from build123d import *

# Parameters (mm, degrees)
F0_R     = 4.5
F1_DEPTH = 7.62
F3_DEPTH = 7.62


with BuildPart() as f1:
    # F0 (on Top) → F1 (new body)
    with BuildSketch(Plane.XY):
        Polygon((-46.3863605133, -12.5119441933), (30.6131504527, -12.5119441933), (41.8083587594, -12.5119441933), (41.8083587594, 80.9429615394), (21.555083004, 80.9429615394), (-37.3282930646, 80.9429615394), (-57.58156882, 80.9429615394), (-57.58156882, -12.5119441933), align=None)
        with Locations((-42.3521250486, -5.9729921632)):
            Circle(F0_R, mode=Mode.SUBTRACT)
        Polygon((-27.3236659841, -8.2207562408), (-15.2949382399, -5.5129789378), (-0.4782718207, -5.5129789378), (11.5504559235, -8.2207562408), align=None, mode=Mode.SUBTRACT)
        with Locations((26.578914988, -5.9729921632)):
            Circle(F0_R, mode=Mode.SUBTRACT)
        Polygon((-25.793466622, 41.4102652967), (-25.793466622, 19.9220313867), (-53.3758333607, -8.2207562408), (-53.3758333607, 76.8635385285), (-25.793466622, 50.1095634738), align=None, mode=Mode.SUBTRACT)
        with Locations((-42.3521250486, 75.2675160766)):
            Circle(F0_R, mode=Mode.SUBTRACT)
        Polygon((-31.369628484, 76.8635385285), (15.5964184234, 76.8635385285), (-7.8866050303, 60.7865828711), align=None, mode=Mode.SUBTRACT)
        Polygon((37.6026233001, -8.2207562408), (10.0202565614, 19.9220313867), (10.0202565614, 41.4102652967), (10.0202565614, 50.1095634738), (37.6026233001, 76.8635385285), align=None, mode=Mode.SUBTRACT)
        with Locations((26.578914988, 75.2675160766)):
            Circle(F0_R, mode=Mode.SUBTRACT)
    extrude(amount=F1_DEPTH)

    # F2 (on face) → F3 (join)
    with BuildSketch(Plane.XY.offset(7.62)):
        Polygon((-7.8866050303, 60.7865828711), (-25.793466622, 50.1095634738), (-25.793466622, 19.9220313867), (-25.793466622, 6.6224359907), (-7.8866050303, -5.5129789378), (10.0202565614, 6.6224359907), (10.0202565614, 19.9220313867), (10.0202565614, 50.1095634738), align=None)
        Polygon((-21.9546725898, 45.3533753753), (-7.8866050303, 56.6663203104), (6.1814625292, 45.3533753753), (6.1814625292, 11.3457208499), (-7.8866050303, 0), (-21.9546725898, 11.3457208499), align=None, mode=Mode.SUBTRACT)
    extrude(amount=F3_DEPTH)


solid = f1.part
Geometry: final body of the model. Coordinates: model frame, mm. A direction names the side the tool comes from. Give positions to 0.01 mm unless a question says otherwise; leave off trailing zeros. Order: outer loops, then holes, each group sorted by start corner. A loop starts at its lowest first (then second) coordinate and runs counter-clockwise, first axis right, second up. Notation, with made-up numbers: (-30, -0.5) -> (27, -0.5) arc R10 cw to (27, 18.5) -> close; hole circle Ø2 at (40, -13). An arc over 180 degrees is marked (long way). Put each result on its own line as item: value.
Q1. Section C-C, the plane z = 13.5. Return loops of the section in (x, y).
Here are the results:
outline: (-25.79, 6.62) -> (-7.89, -5.51) -> (10.02, 6.62) -> (10.02, 50.11) -> (-7.89, 60.79) -> (-25.79, 50.11) -> close; hole (-21.95, 11.35) -> (-7.89, 0) -> (6.18, 11.35) -> (6.18, 45.35) -> (-7.89, 56.67) -> (-21.95, 45.35) -> close
Q2. Section D-D, the plane x = -13. Return loops of the section in (y, z), then the cut area to 3 significant figures.
Here are the results:
outline: (-12.51, 0) -> (-8.22, 0) -> (-8.22, 7.62) -> (-12.51, 7.62) -> close; (-5.51, 0) -> (64.29, 0) -> (64.29, 7.62) -> (57.74, 7.62) -> (57.74, 15.24) -> (52.55, 15.24) -> (52.55, 7.62) -> (4.12, 7.62) -> (4.12, 15.24) -> (-2.05, 15.24) -> (-2.05, 7.62) -> (-5.51, 7.62) -> close; (76.86, 0) -> (80.94, 0) -> (80.94, 7.62) -> (76.86, 7.62) -> close
area: 682 mm^2
Q3. Reachability of faces 1 (the face through (6.181, 29, 11)), 2 (the face through (0.94, 0.47, 11.38)), 3 (the face through (41.808, 34, 4)), 4 (the face through (-19.46, 68.71, 3.76)) from +Z, -Z, +X, -X, +Y, -Y: full face, straight path, thin tool, end or side. Return the list, or none.
Here are the results:
face 1: +Z
face 2: +Z, +X, -Y
face 3: +Z, -Z, +X, +Y, -Y
face 4: +Z, -Z
Q4. Draft query along X for faces 5 (the face through (-7, 80.943, 4)), 6 (the face through (-16.715, 55.523, 11.377)), 7 (the face through (37.603, 35, 4)), 8 (the face through (-53.376, 34, 4)). Return one class per face: released by +X, released by -X, zero draft, split by the parting line, or undercut.
Here are the results:
face 5: zero draft
face 6: released by -X
face 7: undercut
face 8: undercut
Q5. Pin query (flat end, axial travel): pin 1 (11.5 mm diameter, centred on x = -42.35, y = 75.27, fed in from +Z); pin 2 (5.5 mm diameter, centred on x = -42.35, y = -5.97, fed in from -Z); pin 3 (1 mm diameter, centred on x = -10, z = 9.5, fed in from -Y); pin 4 (8.5 mm diameter, centred on y = 33.5, z = 12, fed in from +X). Return the tip coordinate at first contact, or that it passes through.
Here are the results:
pin 1: stops at z = 7.62
pin 2: passes through
pin 3: stops at y = -4.42
pin 4: stops at x = 10.02
Q6. Section A-A, the plane y = 43.5. Return loops of the section in (x, z), then the cut area to 4 significant figures.
Here are the results:
outline: (-57.58, 0) -> (-53.38, 0) -> (-53.38, 7.62) -> (-57.58, 7.62) -> close; (-25.79, 0) -> (10.02, 0) -> (10.02, 15.24) -> (6.18, 15.24) -> (6.18, 7.62) -> (-21.95, 7.62) -> (-21.95, 15.24) -> (-25.79, 15.24) -> close; (37.6, 0) -> (41.81, 0) -> (41.81, 7.62) -> (37.6, 7.62) -> close
area: 395.5 mm^2
Q7. Material intervals for L1, parallel to X at y = 22, z = 3.75; L2, parallel to X at y = 12, z = 1; L3, parallel to X at y = 33.5, z = 12.5, sorted ascending.
Here are the results:
L1: x = -57.58 to -53.38, -25.79 to 10.02, 37.6 to 41.81
L2: x = -57.58 to -53.38, -33.56 to 17.78, 37.6 to 41.81
L3: x = -25.79 to -21.95, 6.18 to 10.02
Q8. Section B-B, the plane x = 18.5. Return loops of the section in (y, z), then the cut area to 3 significant figures.
Here are the results:
outline: (-12.51, 0) -> (11.27, 0) -> (11.27, 7.62) -> (-12.51, 7.62) -> close; (58.33, 0) -> (80.94, 0) -> (80.94, 7.62) -> (58.33, 7.62) -> close
area: 353 mm^2
